Can you work these out from the model? Positions are in its coordinate system, mm. A direction names the side the tool comes from. Coordinates: 2 decimals unless noted, no trailing zeros. Order: outer loops, then holes, each group sorted by start corner. A loop starts at its lowest first (then second) coordinate and runs counter-clockwise, first axis right, second up. Notation, with made-up numbers: (-5, -14.5) -> (6, -14.5) arc R19 cw to (6, -1.5) -> close; hole circle Ø6 at (88.5, 79). An arc over 180 degrees is marked (long way). Answer as a JSON object with one key per item and string values. Group by question number.
(1) I need wall thicknesses on line 1 (X direction, y = -15.25, z = -3). Which ranges of the line are inside material? Lowest first, please.
(2) For pin 1 (10.5 mm diameter, centred on x = 226.5, y = -9.5, fed in from +Z); pin 2 (20.5 mm diameter, centred on x = -227, z = -32.5, fed in from -Y); pin 3 (1.5 mm diameter, centred on x = 85, z = -28, fed in from +Y); pin 4 (20.5 mm diameter, centred on x = 228, z = -41.5, fed in from +Y), each with a flat end and sliding along its axis, tell me the tip position at first contact or that it passes through.
(3) I want a section at B-B, the plane z = -28. List the corners of the cut face in (x, y) for me, plus the area to 3 significant figures.
(4) I want a section at A-A, the plane y = -8.25. List the corners of the cut face in (x, z) for me.
(5) Which directions (+Z, -Z, +X, -X, +Y, -Y) give clear straight access to the entire face, cutting with the end or side of a thin tool? Please do faces 1 (the flat face through (-222, -9, -57.15)), 2 (the flat face through (-222, -14.288, -32)), 3 (the flat face through (222, -4.762, -32)), 4 (the flat face through (-222, -4.762, -32)), 5 (the flat face through (-222, -9, -6.35)).
from build123d import *

# Parameters (mm, degrees)
F0_W     = 419.1
F0_H     = 63.5
F1_DEPTH = 19.05
F2_W     = 9.525
F2_H     = 50.8
F3_DEPTH = 25.4
F4_W     = 9.525
F4_H     = 50.8
F5_DEPTH = 25.4


with BuildPart() as f1:
    # F0 (on Front) → F1 (new body)
    with BuildSketch(Plane.XZ):
        with Locations((0, -31.75)):
            Rectangle(F0_W, F0_H)
    extrude(amount=F1_DEPTH)

    # F2 (on face) → F3 (join)
    with BuildSketch(Plane.YZ.offset(209.55)):
        with Locations((-9.525, -31.75)):
            Rectangle(F2_W, F2_H)
    extrude(amount=F3_DEPTH)

    # F4 (on face) → F5 (join)
    with BuildSketch(Plane(origin=(-209.55, 0, 0), x_dir=(0, -1, 0), z_dir=(-1, 0, 0))):
        with Locations((9.525, -31.75)):
            Rectangle(F4_W, F4_H)
    extrude(amount=F5_DEPTH)


solid = f1.part
Computed values:
{
 "1": {"line 1": "x = -209.55 to 209.55"},
 "2": {"pin 1": "stops at z = -6.35", "pin 2": "stops at y = -14.29", "pin 3": "stops at y = 0", "pin 4": "stops at y = -4.76"},
 "3": {"outline": "(-234.95, -14.29) -> (-209.55, -14.29) -> (-209.55, -19.05) -> (209.55, -19.05) -> (209.55, -14.29) -> (234.95, -14.29) -> (234.95, -4.76) -> (209.55, -4.76) -> (209.55, 0) -> (-209.55, 0) -> (-209.55, -4.76) -> (-234.95, -4.76) -> close", "area": "8,470 mm2"},
 "4": {"outline": "(-234.95, -57.15) -> (-209.55, -57.15) -> (-209.55, -63.5) -> (209.55, -63.5) -> (209.55, -57.15) -> (234.95, -57.15) -> (234.95, -6.35) -> (209.55, -6.35) -> (209.55, 0) -> (-209.55, 0) -> (-209.55, -6.35) -> (-234.95, -6.35) -> close"},
 "5": {"face 1": "-Z, -X, +Y, -Y", "face 2": "+Z, -Z, -X, -Y", "face 3": "+Z, -Z, +X, +Y", "face 4": "+Z, -Z, -X, +Y", "face 5": "+Z, -X, +Y, -Y"}
}
